from build123d import *

# Parameters (mm, degrees)
PAD002_DEPTH      = 10
PAD003_DEPTH      = 10
FILLET_R          = 2.5
BOX013_W          = 42
BOX013_H          = 20
BOX013_DEPTH      = 20
CYLINDER009_R     = 12
CYLINDER009_DEPTH = 10
CYLINDER010_R     = 5
CYLINDER010_DEPTH = 4
CYLINDER011_R     = 3.25
CYLINDER011_DEPTH = 10
CYLINDER012_R     = 2
CYLINDER012_DEPTH = 10
CYLINDER013_R     = 2
CYLINDER013_DEPTH = 10
CYLINDER014_R     = 3
CYLINDER014_DEPTH = 4
CYLINDER015_R     = 3
CYLINDER015_DEPTH = 4
BOX014_W          = 83
BOX014_H          = 10
BOX014_DEPTH      = 10
BOX015_W          = 60
BOX015_H          = 30
BOX015_DEPTH      = 10
BOX016_W          = 65
BOX016_H          = 62
BOX016_DEPTH      = 10
BOX017_W          = 47
BOX017_H          = 23
BOX017_DEPTH      = 5
BOX018_W          = 46
BOX018_H          = 40
BOX018_DEPTH      = 5
BOX019_W          = 65
BOX019_H          = 22
BOX019_DEPTH      = 10
FILLET001_R       = 33
POCKET_DEPTH      = 10


with BuildPart() as part:
    # Sketch012 → Pad002 (new body)
    with BuildSketch(Plane.XY):
        with BuildLine():
            Line((-53.81, 92.96), (46.19, 92.96))
            Line((46.19, 17), (46.19, 92.96))
            Line((38.19, 17), (46.19, 17))
            ThreePointArc((38.19, 17), (-1.06, 29.559572), (-40.31, 17))
            Line((-73.81, 17), (-40.31, 17))
            Line((-73.81, 72), (-73.81, 17))
            ThreePointArc((-53.81, 92.96), (-66.759872, 85.294763), (-73.81, 72))
        make_face()
    extrude(amount=PAD002_DEPTH)

    # Sketch013 (on Face9 of Pad002) → Pad003 (join)
    with BuildSketch(Plane.XY.offset(10)):
        with BuildLine():
            ThreePointArc((38.19, 17), (-0.906062, 29.351664), (-40, 16.993281))
            Line((-40, 20.493281), (-40, 16.993281))
            ThreePointArc((38.19, 20.5), (-0.906031, 32.489323), (-40, 20.493281))
            Line((38.19, 20.5), (38.19, 17))
        make_face()
    extrude(amount=PAD003_DEPTH)

    # Fillet
    fillet_edges = [part.edges().sort_by_distance(p)[0] for p in [
        (-0.906062, 29.351664, 20),
    ]]
    fillet(fillet_edges, radius=FILLET_R)

    # Box013 → Box013 (cut)
    with BuildSketch(Plane(origin=(-74, 13, 0), x_dir=(1, 0, 0), z_dir=(0, 0, 1))):
        with Locations((21, 10)):
            Rectangle(BOX013_W, BOX013_H)
    extrude(amount=BOX013_DEPTH, mode=Mode.SUBTRACT)

    # Cylinder009 → Cylinder009 (cut)
    with BuildSketch(Plane(origin=(4, 90, 0), x_dir=(1, 0, 0), z_dir=(0, 0, 1))):
        Circle(CYLINDER009_R)
    extrude(amount=CYLINDER009_DEPTH, mode=Mode.SUBTRACT)

    # Cylinder010 → Cylinder010 (cut)
    with BuildSketch(Plane(origin=(39, 86, 0), x_dir=(1, 0, 0), z_dir=(0, 0, 1))):
        Circle(CYLINDER010_R)
    extrude(amount=CYLINDER010_DEPTH, mode=Mode.SUBTRACT)

    # Cylinder011 → Cylinder011 (cut)
    with BuildSketch(Plane(origin=(39, 86, 0), x_dir=(1, 0, 0), z_dir=(0, 0, 1))):
        Circle(CYLINDER011_R)
    extrude(amount=CYLINDER011_DEPTH, mode=Mode.SUBTRACT)

    # Cylinder012 → Cylinder012 (cut)
    with BuildSketch(Plane(origin=(-43.9, 79.9, 0), x_dir=(1, 0, 0), z_dir=(0, 0, 1))):
        Circle(CYLINDER012_R)
    extrude(amount=CYLINDER012_DEPTH, mode=Mode.SUBTRACT)

    # Cylinder013 → Cylinder013 (cut)
    with BuildSketch(Plane(origin=(-44, 60, 0), x_dir=(1, 0, 0), z_dir=(0, 0, 1))):
        Circle(CYLINDER013_R)
    extrude(amount=CYLINDER013_DEPTH, mode=Mode.SUBTRACT)

    # Cylinder014 → Cylinder014 (cut)
    with BuildSketch(Plane(origin=(-43.9, 79.9, 0), x_dir=(1, 0, 0), z_dir=(0, 0, 1))):
        Circle(CYLINDER014_R)
    extrude(amount=CYLINDER014_DEPTH, mode=Mode.SUBTRACT)

    # Cylinder015 → Cylinder015 (cut)
    with BuildSketch(Plane(origin=(-44, 60, 0), x_dir=(1, 0, 0), z_dir=(0, 0, 1))):
        Circle(CYLINDER015_R)
    extrude(amount=CYLINDER015_DEPTH, mode=Mode.SUBTRACT)

    # Box014 → Box014 (cut)
    with BuildSketch(Plane(origin=(47.85, 13, 0), x_dir=(0.104528, 0.994522, 0), z_dir=(0, 0, 1))):
        with Locations((41.5, 5)):
            Rectangle(BOX014_W, BOX014_H)
    extrude(amount=BOX014_DEPTH, mode=Mode.SUBTRACT)

    # Box015 → Box015 (cut)
    with BuildSketch(Plane(origin=(-25, 40, 0), x_dir=(1, 0, 0), z_dir=(0, 0, 1))):
        with Locations((30, 15)):
            Rectangle(BOX015_W, BOX015_H)
    extrude(amount=BOX015_DEPTH, mode=Mode.SUBTRACT)

    # Box016 → Box016 (cut)
    with BuildSketch(Plane(origin=(-31, 33, 5), x_dir=(1, 0, 0), z_dir=(0, 0, 1))):
        with Locations((32.5, 31)):
            Rectangle(BOX016_W, BOX016_H)
    extrude(amount=BOX016_DEPTH, mode=Mode.SUBTRACT)

    # Box017 → Box017 (cut)
    with BuildSketch(Plane(origin=(-57, 10, 5), x_dir=(0.829038, 0.559193, 0), z_dir=(0, 0, 1))):
        with Locations((23.5, 11.5)):
            Rectangle(BOX017_W, BOX017_H)
    extrude(amount=BOX017_DEPTH, mode=Mode.SUBTRACT)

    # Box018 → Box018 (cut)
    with BuildSketch(Plane(origin=(43, 19, 5), x_dir=(0.529919, 0.848048, 0), z_dir=(0, 0, 1))):
        with Locations((23, 20)):
            Rectangle(BOX018_W, BOX018_H)
    extrude(amount=BOX018_DEPTH, mode=Mode.SUBTRACT)

    # Box019 → Box019 (cut)
    with BuildSketch(Plane(origin=(-31, 75, 5), x_dir=(1, 0, 0), z_dir=(0, 0.190809, 0.981627))):
        with Locations((32.5, 11)):
            Rectangle(BOX019_W, BOX019_H)
    extrude(amount=BOX019_DEPTH, mode=Mode.SUBTRACT)

    # Fillet001
    fillet001_edges = [part.edges().sort_by_distance(p)[0] for p in [
        (-31, 55.280234, 7.5),
    ]]
    fillet(fillet001_edges, radius=FILLET001_R)

    # Sketch015 (on Face8 of Fillet001) → Pocket (cut)
    with BuildSketch(Plane(origin=(-31, 75, 10), x_dir=(1, 0, 0), z_dir=(0, 0, 1))):
        with BuildLine():
            ThreePointArc((-16.55, -13), (-30.9, -19.166644), (-16.55, -25.333288))
            Line((-16.55, -13), (-16.55, -25.333288))
        make_face()
    extrude(amount=-POCKET_DEPTH, mode=Mode.SUBTRACT)


solid = part.part
CAD build for the part. Positions are in the model's coordinates, mm. A direction names the side the tool comes from. Coordinates: 2 decimals unless noted, no trailing zeros. Loops run counter-clockwise (first coordinate to the right, second up) from the corner with the lowest first, then second, coordinate; pieces in that order, holes last. Notation, with made-up numbers: (52.25, 1) - (89.25, 1) arc R19 ccw to (89.25, 37) - close; hole circle Ø9 at (71.25, -29). An arc over 180 degrees is marked (long way). Write item = value, one per line. Start each with the question number.
Q1. Flat gauge pins, fed straight in: pin 1 Ø8 at (x, z) = (-28.5, 17) entering from +Y; pin 2 Ø2.5 at (x, z) = (4.5, 8) entering from +Y; pin 3 Ø4 at (y, z) = (27.5, 3) entering from +X. Where does each tip first touch, or does it go through?
Q2. Drill centre lines: L1, parallel to Y at x = -43.9, z = 2.4; L2, parallel to X at y = 79.9, z = 8.05; L3, parallel to X at y = 86, z = 8.1. Where is each one in solid material? Low to high.
Q3. Pull direction X, two halves, no side cores. Call faces 1 (the cylindrical face through (-44.334, 77.948, 6.958)), 2 (the flat face through (29.78, 27.26, 7.46)), 3 (the flat face through (3, 32, 20)): pulls with the +X half, pulls with the -X half, needs draft (parallel to the pull), parting line crosses it, or undercut.
Q4. Cut at A-A, the plane z = 8. Give the number of separate pieces and of enclosed holes in the cut face, then the cut area to 3 significant figures.
Q5. Which spindle directions (+Z, -Z, +X, -X, +Y, -Y) get a long thin tool onto all of the face, cutting with end or side? Do faces 4 (the flat face through (-58, 33, 4)), 5 (the flat face through (-54.919, 39.147, 7.465)), 6 (the flat face through (-42, 81, 4)), 7 (the flat face through (-31, 83, 7)), 8 (the flat face through (-25, 55, 2)). Say none if no direction does.
Q6. Cut at B-B, the plane x = -51. List the corners of the cut face in (y, z), then the cut area to 3 significant figures.
Q7. Cut at C-C, the plane y = 67.5. List the corners of the cut face in (x, z).
Computed:
q1.pin_1 = 28.37
q1.pin_2 = 33
q1.pin_3 = 39.53
q2.L1 = 33 to 57, 63 to 76.9, 82.9 to 92.96
q2.L2 = -70.78 to -45.9, -41.9 to -31, 34 to 44.83
q2.L3 = -66.06 to -31, 34 to 35.75, 42.25 to 45.47
q3.face_1 = undercut
q3.face_2 = pulls with the +X half
q3.face_3 = needs draft
q4.separate_pieces = 3
q4.enclosed_holes = 4
q4.area = 2,310 mm²
q5.face_4 = +Z, -Z, -X, -Y
q5.face_5 = +Z, +X, -Y
q5.face_6 = -Z
q5.face_7 = +Z, +Y
q5.face_8 = +Z, -Z
q6.outline = (33, 0) - (47.68, 0) - (47.68, 10) - (41.79, 10) - (41.79, 5) - (33, 5) - close; (63.99, 0) - (92.96, 0) - (92.96, 10) - (63.99, 10) - close
q6.area = 393 mm²
q7.outline = (-73.81, 0) - (-25, 0) - (-25, 5) - (-31.43, 5) - (-31.43, 10) - (-73.81, 10) - close; (35, 0) - (43.52, 0) - (43.52, 5) - (35, 5) - close
